CAD build for the part. Positions are in the model's coordinates, mm. A direction names the side the tool comes from. Coordinates: 2 decimals unless noted, no trailing zeros. Loops run counter-clockwise (first coordinate to the right, second up) from the corner with the lowest first, then second, coordinate; pieces in that order, holes last. Notation, with made-up numbers: (-9.5, -7) -> (3.5, -7) arc R25 cw to (3.5, 16) -> close; hole circle Ø3 at (-32.75, -28.5). An arc over 180 degrees is marked (long way). Write item = value, one per line. Start each with the question number.
(1) Band-saw the part on C-C (y = -4.5). Write the cut outline in (x, z) (3 decimals), and give its area (3 significant figures).
(2) Drill centre lines: line 1 (Z direction, x = 2.5, y = 0); line 2 (Z direction, x = 2.95, y = 3.5); line 3 (Z direction, x = 0.95, y = 7). Where is each one in solid material? Low to high. Write a range as from..to.
(3) Band-saw the part on A-A (y = 6.25). Write the cut outline in (x, z) (3 decimals), and give its area (3 significant figures).
(4) Tool access for faces 1 (the face through (2, -6, -6.095)), 2 (the face through (3.175, -4, 1)), 3 (the face through (2, -6, 7.01)): list every direction of +Z, -Z, +X, -X, +Y, -Y with a clear straight run to the whole face (end or side of a thin tool).
(5) Pull direction Z, two halves, no side cores. Call faces 4 (the face through (2, -12.967, 1)), 5 (the face through (1.57, 1.69, 0.2)), 6 (the face through (1.565, 6.001, -7.468)): +Z half, -Z half, draft (parallel to the pull), parting line (faces both ways), or undercut.
(6) Flat gauge pin, fed straight in: P1, Ø1, axis at x = 1, y = 3.5, coming from the +Z side. Where does the tip first touch, or does it go through?
(7) Band-saw the part on D-D (z = -2.5). Write the cut outline in (x, y) (3 decimals).
(8) Band-saw the part on B-B (x = 1.85). Write the cut outline in (y, z).
```python
from build123d import *

# Parameters (mm, degrees)
F1_DEPTH = 3.175


# Not quite as in the source:
# - a feature names something its author has since deleted; it is built from what else it names


with BuildPart() as f1:
    # F0 (on Right) → F1 (new body)
    with BuildSketch(Plane.YZ):
        with BuildLine():
            Line((-0.0335522907, 7.0097496485), (-12.9674749849, 7.0097496485))
            Line((-12.9674749849, 7.0097496485), (-12.9674749849, -6.0952282245))
            Line((-12.9674749849, -6.0952282245), (0.1951931324, -6.0952282245))
            ThreePointArc((0.1951931324, -6.0952282245), (1.3039147966, -6.2365574954), (2.3417274082, -6.651506498))
            ThreePointArc((2.3417274082, -6.651506498), (6.055282807, -7.4637663122), (9.6017406465, -6.0952282245))
            Line((9.6017406465, -6.0952282245), (9.6017406465, -4.4064043338))
            ThreePointArc((9.6017406465, -4.4064043338), (1.6888526066, 0.3560956662), (9.6017406465, 5.1185956662))
            Line((9.6017406465, 5.1185956662), (9.6017406465, 7.0097496485))
            ThreePointArc((9.6017406465, 7.0097496485), (5.9747824086, 8.4525130692), (2.1664773001, 7.5962394284))
            ThreePointArc((2.1664773001, 7.5962394284), (1.1048786978, 7.158888427), (-0.0335522907, 7.0097496485))
        make_face()
    extrude(amount=F1_DEPTH)


solid = f1.part
```
Findings below:
q1.outline = (0, -6.095) -> (3.175, -6.095) -> (3.175, 7.01) -> (0, 7.01) -> close
q1.area = 41.6 mm²
q2.line_1 = -6.1..7.01
q2.line_2 = -7.16..-3.67, 4.39..8.18
q2.line_3 = -7.32..-5.03, 5.75..8.29
q3.outline = (0, -7.446) -> (3.175, -7.446) -> (3.175, -4.969) -> (0, -4.969) -> close; (0, 5.682) -> (3.175, 5.682) -> (3.175, 8.425) -> (0, 8.425) -> close
q3.area = 16.6 mm²
q4.face_1 = -Z, +X, -X, -Y
q4.face_2 = +Z, -Z, +X, +Y, -Y
q4.face_3 = +Z, +X, -X, -Y
q5.face_4 = draft
q5.face_5 = undercut
q5.face_6 = -Z half
q6.P1 = 8.31
q7.outline = (0, -12.967) -> (3.175, -12.967) -> (3.175, 2.508) -> (0, 2.508) -> close
q8.outline = (-12.97, -6.1) -> (0.2, -6.1) arc R4.42 cw to (2.34, -6.65) arc R6.61 ccw to (9.6, -6.1) -> (9.6, -4.41) arc R5.39 cw (long way) to (9.6, 5.12) -> (9.6, 7.01) arc R6.61 ccw to (2.17, 7.6) arc R4.42 cw to (-0.03, 7.01) -> (-12.97, 7.01) -> close
